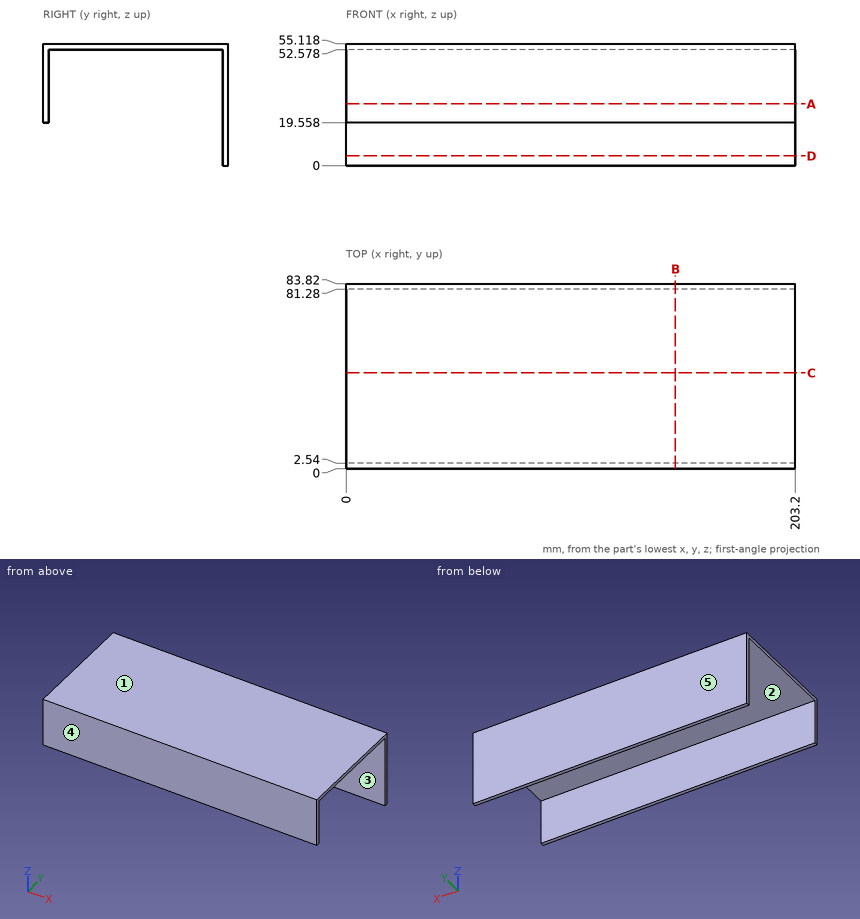
Print and shaded views of the part. All mm, measured from the part's lowest x, y and z. A direction names the side the tool comes from. Give positions to 0.01 mm unless a question says otherwise; leave off trailing zeros. Loops run counter-clockwise (first coordinate to the right, second up) from the corner with the lowest first, then second, coordinate; pieces in that order, holes last. Notation, with made-up numbers: (18.25, 22.5) - (50.25, 22.5) arc R33 ccw to (50.25, 50.5) - close; hole circle Ø2 at (56.5, -5). An arc over 180 degrees is marked (long way). Use a Markdown table: item, result.
(1) Band-saw the part on B-B (x = 149). Give the cut face in (y, z).
Taken from the geometry:
| item | result |
|---|---|
| outline | (0, 19.56) - (2.54, 19.56) - (2.54, 52.58) - (81.28, 52.58) - (81.28, 0) - (83.82, 0) - (83.82, 55.12) - (0, 55.12) - close |
(2) Band-saw the part on D-D (z = 4.5). Give the cut face in (x, y).
Taken from the geometry:
| item | result |
|---|---|
| outline | (0, 81.28) - (203.2, 81.28) - (203.2, 83.82) - (0, 83.82) - close |
(3) Band-saw the part on C-C (y = 43.5). Give the cut face in (x, z), and give its area (3 significant figures).
Taken from the geometry:
| item | result |
|---|---|
| outline | (0, 52.58) - (203.2, 52.58) - (203.2, 55.12) - (0, 55.12) - close |
| area | 516 mm2 |
(4) Pull direction Y, two halves, no side cores. Call the marked faces 3, 4 and 5: +Y half, -Y half, draft (parallel to the pull), parting line (faces both ways), or undercut.
Taken from the geometry:
| item | result |
|---|---|
| face 3 | undercut |
| face 4 | -Y half |
| face 5 | +Y half |
(5) Drop flat-ended pins along their axis: pin 1 Ø0.8 at (x, y) = (131, 1.5) entering from -Z; pin 2 Ø4 at (x, y) = (132.5, 48.5) entering from -Z; pin 3 Ø1.5 at (x, z) = (39.5, 8) entering from -Y. Give the stop position or say it passes through.
Taken from the geometry:
| item | result |
|---|---|
| pin 1 | z = 19.56 |
| pin 2 | z = 52.58 |
| pin 3 | y = 81.28 |
(6) Band-saw the part on A-A (z = 28). Give the cut face in (x, y).
Taken from the geometry:
| item | result |
|---|---|
| outline | (0, 0) - (203.2, 0) - (203.2, 2.54) - (0, 2.54) - close; (0, 81.28) - (203.2, 81.28) - (203.2, 83.82) - (0, 83.82) - close |
(7) Wall check: line 1 along Y through (x, z) = (43.5, 36.5); line 2 along Y through (x, z) = (97, 5.5); line 3 along Z through (x, y) = (96, 31). Give the ranges that are in metal, low to high.
Taken from the geometry:
| item | result |
|---|---|
| line 1 | 0 to 2.54, 81.28 to 83.82 |
| line 2 | 81.28 to 83.82 |
| line 3 | 52.58 to 55.12 |
(8) Which spindle directions (+Z, -Z, +X, -X, +Y, -Y) get a long thin tool onto all of the face, cutting with end or side? Do the marked faces 1 and 2. Say none if no direction does.
Taken from the geometry:
| item | result |
|---|---|
| face 1 | +Z, +X, -X, +Y, -Y |
| face 2 | -Z, +X, -X |
